from build123d import *

# Parameters (mm, degrees)
SKETCH_1_W               = 72
SKETCH_1_H               = 100
EXTRUDE_1_DEPTH          = 3
SKETCH_2_W               = 72
SKETCH_2_H               = 3
EXTRUDE_2_DEPTH          = 24
CUT_EXTRUDE_1_DEPTH      = 83.346827504
CUT_EXTRUDE_1_DEPTH_BACK = 83.346827504
SKETCH_3_W               = 3
SKETCH_3_H               = 50
CUT_EXTRUDE_2_DEPTH      = 83.346827504
CUT_EXTRUDE_2_DEPTH_BACK = 83.346827504
SKETCH_5_R               = 1.75
CUT_EXTRUDE_3_DEPTH      = 83.346827504
CUT_EXTRUDE_3_DEPTH_BACK = 83.346827504
SKETCH_6_R               = 1.75
FILLET_1_R               = 5
FILLET_2_R               = 2
CUT_EXTRUDE_5_DEPTH      = 83.346827504
CUT_EXTRUDE_5_DEPTH_BACK = 83.346827504
SKETCH_8_R               = 1.75


with BuildPart() as part:
    # 草图1 → 凸台-拉伸1 (new body)
    with BuildSketch(Plane(origin=(0, 0, 0), x_dir=(1, 0, 0), z_dir=(0, 1, 0))):
        Rectangle(SKETCH_1_W, SKETCH_1_H)
    extrude(amount=EXTRUDE_1_DEPTH)

    # 草图2 → 凸台-拉伸2 (add)
    with BuildSketch(Plane.XY.offset(50)):
        with Locations((0, 1.5)):
            Rectangle(SKETCH_2_W, SKETCH_2_H)
    extrude(amount=EXTRUDE_2_DEPTH)

    # 草图3 → 切除-拉伸1 (cut, two sides: drawn at the far end of the back side and taken through both)
    with BuildSketch(Plane(origin=(0, 3, 0), x_dir=(1, 0, 0), z_dir=(0, 1, 0)).offset(-CUT_EXTRUDE_1_DEPTH_BACK)):
        with Locations((-34.5, 25)):
            Rectangle(SKETCH_3_W, SKETCH_3_H)
        with Locations((34.5, 25)):
            Rectangle(SKETCH_3_W, SKETCH_3_H)
        with Locations((-34.5, -49)):
            Rectangle(SKETCH_3_W, SKETCH_3_H)
        with Locations((34.5, -49)):
            Rectangle(SKETCH_3_W, SKETCH_3_H)
    extrude(amount=CUT_EXTRUDE_1_DEPTH + CUT_EXTRUDE_1_DEPTH_BACK, mode=Mode.SUBTRACT)

    # 草图5 → 切除-拉伸2 (cut, two sides: drawn at the far end of the back side and taken through both)
    with BuildSketch(Plane(origin=(0, 3, 0), x_dir=(1, 0, 0), z_dir=(0, 1, 0)).offset(-CUT_EXTRUDE_2_DEPTH_BACK)):
        with Locations(Location((-23.5, 40.5, 0), (0, 0, 270))):
            Circle(SKETCH_5_R)
    extrude(amount=CUT_EXTRUDE_2_DEPTH + CUT_EXTRUDE_2_DEPTH_BACK, mode=Mode.SUBTRACT)

    # 草图6 → 切除-拉伸3 (cut, two sides: drawn at the far end of the back side and taken through both)
    with BuildSketch(Plane(origin=(0, 3, 0), x_dir=(1, 0, 0), z_dir=(0, 1, 0)).offset(-CUT_EXTRUDE_3_DEPTH_BACK)):
        with Locations(Location((23.5, 40.5, 0), (0, 0, 270))):
            Circle(SKETCH_6_R)
        with Locations(Location((-23.5, -64.5, 0), (0, 0, 270))):
            Circle(SKETCH_6_R)
        with Locations(Location((23.5, -64.5, 0), (0, 0, 270))):
            Circle(SKETCH_6_R)
    extrude(amount=CUT_EXTRUDE_3_DEPTH + CUT_EXTRUDE_3_DEPTH_BACK, mode=Mode.SUBTRACT)

    # 圆角1
    fillet_1_edges = [part.edges().sort_by_distance(p)[0] for p in [
        (33, 1.5, -50),
        (-33, 1.5, 74),
        (33, 1.5, 74),
        (-33, 1.5, -50),
    ]]
    fillet(fillet_1_edges, radius=FILLET_1_R)

    # 圆角2
    fillet_2_edges = [part.edges().sort_by_distance(p)[0] for p in [
        (36, 1.5, 0),
        (-36, 1.5, 24),
        (36, 1.5, 24),
        (-36, 1.5, 0),
    ]]
    fillet(fillet_2_edges, radius=FILLET_2_R)

    # 草图8 → 切除-拉伸5 (cut, two sides: drawn at the far end of the back side and taken through both)
    with BuildSketch(Plane(origin=(0, 3, 0), x_dir=(1, 0, 0), z_dir=(0, 1, 0)).offset(-CUT_EXTRUDE_5_DEPTH_BACK)):
        with Locations(Location((0, 40.5, 0), (0, 0, 270))):
            Circle(SKETCH_8_R)
        with Locations(Location((0, -64.5, 0), (0, 0, 270))):
            Circle(SKETCH_8_R)
    extrude(amount=CUT_EXTRUDE_5_DEPTH + CUT_EXTRUDE_5_DEPTH_BACK, mode=Mode.SUBTRACT)


solid = part.part
Verification items for the finished model (mm, model axes). A direction names the side the tool comes from. Give positions to 0.01 mm unless a question says otherwise; leave off trailing zeros. Write each loop counter-clockwise with the first axis right and the second up, starting at its lowest first coordinate (ties: lowest second). Pieces come first, ordered by that corner, then holes.
(1) Cross-section at C-C (y = 1.95). Enter the section's corners in (x, z), plus the area to 3 significant figures.
(2) Cross-section at D-D (z = 64). Enter the section's corners in (x, y).
(3) Mould release check, pull along X, two halves, no side actions. Record for faces 1 (the face through (-1, 0, 11)), 2 (the face through (-36, 1, 12)), 3 (the face through (-22, 1.5, -39.6)): +X half, -X half, draft (parallel to the pull), parting line (faces both ways), or undercut.
(4) Cross-section at B-B (x = -23.5). Enter the section's corners in (y, z).
(5) Access from +Z, -Z, +X, -X, +Y, -Y to the whole of each face (thin tool, end or side, straight path). Record for faces 4 (the face through (33, 1, -22)), 5 (the face through (-33, 1, 47)), 6 (the face through (-33, 1, -22)).
(6) Material ranges on line 1 (X direction, y = 1.15, z = -40.5); line 2 (Z direction, x = 23.5, y = 2.2); line 3 (Z direction, x = -22, y = 0.15), recorded low to high.
(7) Cross-section at A-A (z = -40.5). Enter the section's corners in (x, y).
(8) Gauge pin test, flat ends, axial feed: pin 1 (0.5 mm diameter, centred on x = -33.5, y = 1.5, fed in from +Z); pin 2 (3 mm diameter, centred on x = 23.5, z = 0.5, fed in from -Y); pin 3 (0.8 mm diameter, centred on x = 33.5, y = 1, fed in from -Z); pin 4 (1.5 mm diameter, centred on y = 1, z = -23.5, fed in from +X). Record the tip position at first contact, or that the pin passes through.
Worked out:
1. outline: (-36, 2) arc R2 ccw to (-34, 0) - (-33, 0) - (-33, -45) arc R5 ccw to (-28, -50) - (28, -50) arc R5 ccw to (33, -45) - (33, 0) - (34, 0) arc R2 ccw to (36, 2) - (36, 22) arc R2 ccw to (34, 24) - (33, 24) - (33, 69) arc R5 ccw to (28, 74) - (-28, 74) arc R5 ccw to (-33, 69) - (-33, 24) - (-34, 24) arc R2 ccw to (-36, 22) - close; hole circle Ø3.5 at (-23.5, -40.5); hole circle Ø3.5 at (-23.5, 64.5); hole circle Ø3.5 at (0, -40.5); hole circle Ø3.5 at (0, 64.5); hole circle Ø3.5 at (23.5, -40.5); hole circle Ø3.5 at (23.5, 64.5)
1. area: 8,250 mm2
2. outline: (-33, 0) - (-25.18, 0) - (-25.18, 3) - (-33, 3) - close; (-21.82, 0) - (-1.68, 0) - (-1.68, 3) - (-21.82, 3) - close; (1.68, 0) - (21.82, 0) - (21.82, 3) - (1.68, 3) - close; (25.18, 0) - (33, 0) - (33, 3) - (25.18, 3) - close
3. face 1: draft
3. face 2: -X half
3. face 3: undercut
4. outline: (0, -50) - (3, -50) - (3, -42.25) - (0, -42.25) - close; (0, -38.75) - (3, -38.75) - (3, 62.75) - (0, 62.75) - close; (0, 66.25) - (3, 66.25) - (3, 74) - (0, 74) - close
5. face 4: -Z, +X, +Y, -Y
5. face 5: +Z, -X, +Y, -Y
5. face 6: -Z, -X, +Y, -Y
6. line 1: x = -33 to -25.25, -21.75 to -1.75, 1.75 to 21.75, 25.25 to 33
6. line 2: z = -50 to -42.25, -38.75 to 62.75, 66.25 to 74
6. line 3: z = -50 to -41.4, -39.6 to 63.6, 65.4 to 74
7. outline: (-33, 0) - (-25.25, 0) - (-25.25, 3) - (-33, 3) - close; (-21.75, 0) - (-1.75, 0) - (-1.75, 3) - (-21.75, 3) - close; (1.75, 0) - (21.75, 0) - (21.75, 3) - (1.75, 3) - close; (25.25, 0) - (33, 0) - (33, 3) - (25.25, 3) - close
8. pin 1: stops at z = 24
8. pin 2: stops at y = 0
8. pin 3: stops at z = 0
8. pin 4: stops at x = 33
